```python
from build123d import *

# Parameters (mm, degrees)
SKETCH_1_R          = 21
SKETCH_1_R_2        = 13.5
EXTRUDE_1_DEPTH     = 5.5
SKETCH_2_R          = 1.3
CUT_EXTRUDE_1_DEPTH = 8


with BuildPart() as part:
    # 草图1 → 凸台-拉伸1 (new body)
    with BuildSketch(Plane.XY):
        Circle(SKETCH_1_R)
        Circle(SKETCH_1_R_2, mode=Mode.SUBTRACT)
    extrude(amount=EXTRUDE_1_DEPTH)

    # 草图2 → 切除-拉伸1 (cut)
    with BuildSketch(Plane(origin=(0, 0, 0), x_dir=(-1, 0, 0), z_dir=(0, 0, -1))):
        with Locations((-12.374368671, 12.374368671)):
            Circle(SKETCH_2_R)
        with Locations((12.374368671, 12.374368671)):
            Circle(SKETCH_2_R)
        with Locations((12.374368671, -12.374368671)):
            Circle(SKETCH_2_R)
        with Locations((-12.374368671, -12.374368671)):
            Circle(SKETCH_2_R)
    extrude(amount=-CUT_EXTRUDE_1_DEPTH, mode=Mode.SUBTRACT)


solid = part.part
```
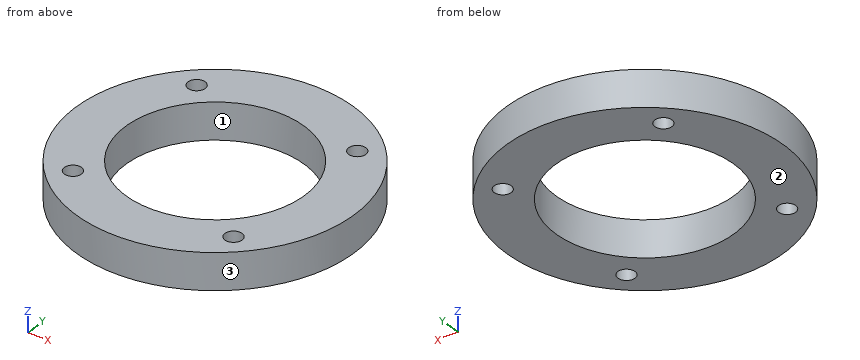
Part model, mm, in its own coordinate system. Face numbers are marked on the shaded views. Round coordinates to 2 decimals unless told otherwise and drop trailing zeros. Loops run counter-clockwise (first coordinate to the right, second up) from the corner with the lowest first, then second, coordinate; pieces in that order, holes last.
Item 1: Drill centre lines: line 1 (Y direction, x = 0, z = 4.2); line 2 (Y direction, x = 4, z = 4.75); line 3 (X direction, y = -3, z = 0.7). Where is each one in solid material? Low to high.
Item 2: Mould opens along Y. For the marked faces 1, 2 and 3 say: +Y half, -Y half, draft (parallel to the pull), parting line (faces both ways), or undercut.
Item 3: Cut at D-D, the plane y = -15.5. Give the cut face in (x, z).
Item 4: Cut at C-C, the plane z = 2.6. Give the cut face in (x, y), then the cut area to 3 significant figures.
Item 5: Cut at A-A, the plane x = 0. Give the cut face in (y, z).
Item 6: Drop flat-ended pins along their axis: P1, Ø1.6, axis at x = 12.37, y = -12.37, coming from the +Z side; P2, Ø3, axis at x = -12.37, y = 12.37, coming from the +Z side; P3, Ø1, axis at x = 13, z = 1, coming from the -Y side; P4, Ø2, axis at y = 14, z = 1, coming from the -X side. Give the stop position or say it passes through.
A:
1. line 1: y = -21 to -13.5, 13.5 to 21
1. line 2: y = -20.62 to -12.89, 12.89 to 20.62
1. line 3: x = -20.78 to -13.16, 13.16 to 20.78
2. face 1: undercut
2. face 2: draft
2. face 3: parting line
3. outline: (-14.17, 0) - (14.17, 0) - (14.17, 5.5) - (-14.17, 5.5) - close
4. outline: circle Ø42 at (0, 0); hole circle Ø2.6 at (-12.37, -12.37); hole circle Ø2.6 at (-12.37, 12.37); hole circle Ø27 at (0, 0); hole circle Ø2.6 at (12.37, -12.37); hole circle Ø2.6 at (12.37, 12.37)
4. area: 792 mm2
5. outline: (-21, 0) - (-13.5, 0) - (-13.5, 5.5) - (-21, 5.5) - close; (13.5, 0) - (21, 0) - (21, 5.5) - (13.5, 5.5) - close
6. P1: passes through
6. P2: stops at z = 5.5
6. P3: stops at y = -16.87
6. P4: stops at x = -16.49
